For this review, take the finished solid that the model builds, in its own axes (mm). A direction names the side the tool comes from. Coordinates: 2 decimals unless noted, no trailing zeros. Order: outer loops, then holes, each group sorted by start corner. A loop starts at its lowest first (then second) coordinate and runs counter-clockwise, first axis right, second up. Notation, with made-up numbers: M 24.25,8 L 66.25,8 A13 cw 66.25,26 Z; hole C 32,58.25 d7. An arc over 180 degrees is marked long. Use CSV: the item, a comma, the result in double quotes.
```python
from build123d import *

# Parameters (mm, degrees)
F1_DEPTH = 19.05
F2_W     = 19.05
F2_H     = 152.4
F2_W_2   = 152.4
F2_H_2   = 38.1
F3_DEPTH = 19.05


# Not quite as in the source:
# - a length typed as a fraction of an inch, garbled in the dataset ("3 / 203.2 mm" for 3/8 in), is restored


with BuildPart() as f1:
    # F0 (on Right) → F1 (new body)
    with BuildSketch(Plane.YZ):
        Polygon((-127, 50.8), (-381, 50.8), (-381, -425.45), (381, -425.45), (381, 508), (-127, 508), align=None)
    extrude(amount=F1_DEPTH)

    # F2 (on face) → F3 (cut)
    with BuildSketch(Plane.YZ.offset(19.05)):
        with Locations((371.475, 279.4)):
            Rectangle(F2_W, F2_H)
        with Locations((371.475, -177.8)):
            Rectangle(F2_W, F2_H)
        with Locations((53.975, 431.8)):
            Rectangle(F2_W, F2_H)
        with Locations((-117.475, 279.4)):
            Rectangle(F2_W, F2_H)
        with Locations((212.725, 279.4)):
            Rectangle(F2_W, F2_H)
        with Locations((212.725, -177.8)):
            Rectangle(F2_W, F2_H)
        with Locations((-117.475, -177.8)):
            Rectangle(F2_W, F2_H)
        with Locations((-371.475, -177.8)):
            Rectangle(F2_W, F2_H)
        with Locations((152.4, -406.4)):
            Rectangle(F2_W_2, F2_H_2)
        with Locations((-152.4, -406.4)):
            Rectangle(F2_W_2, F2_H_2)
    extrude(amount=-F3_DEPTH, mode=Mode.SUBTRACT)


solid = f1.part
```
Item 1: Add section B-B on z = -220. State the section outline as (x, y) points, and give its area (3 significant figures).
Solutions:
outline,"M 0,-361.95 L 19.05,-361.95 L 19.05,-127 L 0,-127 Z; M 0,-107.95 L 19.05,-107.95 L 19.05,203.2 L 0,203.2 Z; M 0,222.25 L 19.05,222.25 L 19.05,361.95 L 0,361.95 Z"
area,"13,100 mm^2"
Item 2: For faces 1 (the face through (10, -361.95, -179)), 2 (the face through (10, 44.45, 431)), 3 (the face through (10, 76.2, -407)), 4 (the face through (9, -127, 433)), 5 (the face through (10, -127, -179)), list the 3-axis set-ups (+Z, -Z, +X, -X, +Y, -Y) from which the entire face can be reached by the end or side of a thin tool; tool diameter is ignored.
Solutions:
face 1,"+X, -X, -Y"
face 2,"+Z, +X, -X"
face 3,"-Z, +X, -X"
face 4,"+Z, +X, -X, -Y"
face 5,"+X, -X"
Item 3: Add section C-C on z = 237. State the section outline as (x, y) points.
Solutions:
outline,"M 0,-107.95 L 19.05,-107.95 L 19.05,203.2 L 0,203.2 Z; M 0,222.25 L 19.05,222.25 L 19.05,361.95 L 0,361.95 Z"
Item 4: Add section A-A on z = 404. State the section outline as (x, y) points, and give its area (3 significant figures).
Solutions:
outline,"M 0,-127 L 19.05,-127 L 19.05,44.45 L 0,44.45 Z; M 0,63.5 L 19.05,63.5 L 19.05,381 L 0,381 Z"
area,"9,310 mm^2"
Item 5: Add section D-D on x = 6.25. State how many separate pieces and enclosed holes the cut face has, and give its area (3 significant figures).
Solutions:
separate pieces,"1"
enclosed holes,"3"
area,"560,000 mm^2"
Item 6: Clearance check with flat-ended pins moving along their axes: pin 1 Ø9.5 at (x, y) = (7, -170.5) entering from -Z; pin 2 Ø5.5 at (x, z) = (11, 247.5) entering from -Y; pin 3 Ø9.5 at (x, z) = (8.5, 242) entering from +Y. State where each tip first meets the part, or that it passes through.
Solutions:
pin 1,"z = -387.35"
pin 2,"y = -107.95"
pin 3,"y = 361.95"
Item 7: Draft analysis for pull direction Z (two halves, no side actions). For faces 6 (the face through (10, -76.2, -407)), 7 (the face through (10, 371, -254)), 8 (the face through (9, -252, 50.8)), state which applies: released by +Z, released by -Z, zero draft, split by the parting line, or undercut.
Solutions:
face 6,"zero draft"
face 7,"undercut"
face 8,"released by +Z"
Item 8: To check wall thickness, follow line 1 along Y through (x, z) = (10.25, -146.5); line 2 along Y through (x, z) = (12.75, 449); line 3 along Y through (x, z) = (13, 311.5). State the ranges of each line that lie inside material, in increasing order. Write a range as [from, to].
Solutions:
line 1,"[-361.95, -127], [-107.95, 203.2], [222.25, 361.95]"
line 2,"[-127, 44.45], [63.5, 381]"
line 3,"[-107.95, 203.2], [222.25, 361.95]"
